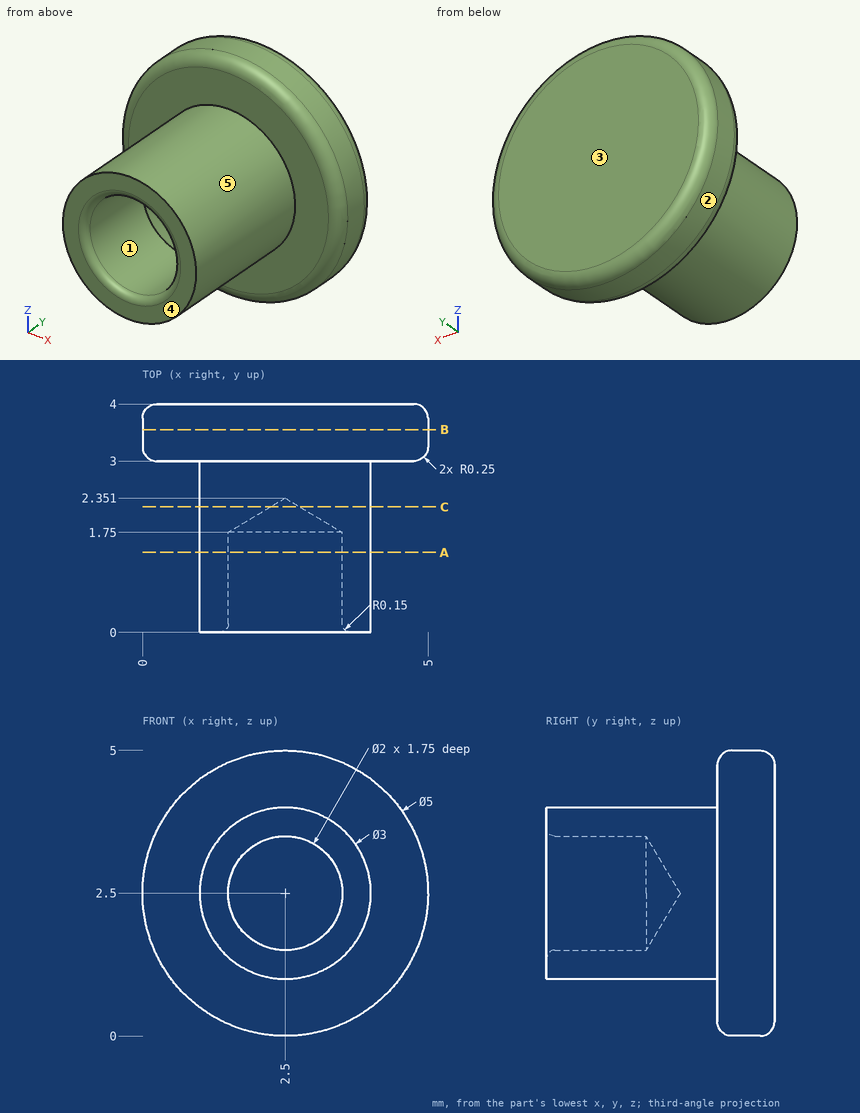
The figure shows three views and two pictorial views of one solid part (mm, origin at its lowest corner). Answer the questions. A direction names the side the tool comes from. Give positions to 0.01 mm unless a question says otherwise; leave off trailing zeros. Loops run counter-clockwise (first coordinate to the right, second up) from the corner with the lowest first, then second, coordinate; pieces in that order, holes last. Notation, with made-up numbers: (-5, -34) -> (34, -34) arc R19 ccw to (34, -21) -> close; hole circle Ø11 at (59, -14). An arc over 180 degrees is marked (long way). Put each result on its own line as item: value. Start each with the question number.
Item 1: Which of the six approach directions +Z, -Z, +X, -X, +Y, -Y give full straight-line access (tool end or side, diameter ignored) to the marked faces 4 and 5?
Item 2: The part is cut by section C-C (y = 2.2). Give the vertices of the cut face in (x, z).
Item 3: The part is cut by section A-A (y = 1.4). Give the vertices of the cut face in (x, z).
Item 4: The part is cut by section B-B (y = 3.55). Give the vertices of the cut face in (x, z).
Item 5: Find the intervals of material crossed by L1, parallel to Y at x = 2.95, z = 0.6; L2, parallel to X at y = 1.7, z = 3.8; L3, parallel to Z at x = 2.4, y = 0.85 (1 decimal), in increasing order. Write a range as [from, to].
Item 6: The mould has two halves that part along Z. Classify the marked faces 1, 2 and 3: released by +Z, released by -Z, zero draft, split by the parting line, or undercut.
Answers below:
1. face 4: +Z, -Z, +X, -X, -Y
1. face 5: -Y
2. outline: circle Ø3 at (2.5, 2.5); hole circle Ø0.5 at (2.5, 2.5)
3. outline: circle Ø3 at (2.5, 2.5); hole circle Ø2 at (2.5, 2.5)
4. outline: circle Ø5 at (2.5, 2.5)
5. L1: [3, 4]
5. L2: [1.75, 3.25]
5. L3: [1, 1.5], [3.5, 4]
6. face 1: undercut
6. face 2: split by the parting line
6. face 3: zero draft
